Can you work these out from the model? Positions are in its coordinate system, mm. A direction names the side the tool comes from. Round coordinates to 2 decimals unless told otherwise and drop trailing zeros. Order: outer loops, then holes, each group sorted by start corner. A loop starts at its lowest first (then second) coordinate and runs counter-clockwise, first axis right, second up.
from build123d import *

# Parameters (mm, degrees)
SKETCH1_W                    = 25
SKETCH1_H                    = 30
BASE_FLANGE1_DEPTH           = 1.5
EDGE_FLANGE1_STRIP_CUT_DEPTH = 25
EDGE_FLANGE1_DEPTH           = 25
EDGE_FLANGE2_STRIP_CUT_DEPTH = 25
EDGE_FLANGE2_DEPTH           = 25
EDGE_FLANGE3_DEPTH           = 10
EDGE_FLANGE4_DEPTH           = 25
EDGE_FLANGE4_BEND_DEPTH      = 25


# Sheet-metal steps are written as plain solids
with BuildPart() as part:
    # Sketch1 → Base-Flange1 (new body)
    with BuildSketch(Plane(origin=(0, 0, 0), x_dir=(0, 0, -1), z_dir=(1, 0, 0))):
        Rectangle(SKETCH1_W, SKETCH1_H)
    extrude(amount=BASE_FLANGE1_DEPTH)

    # Edge-Flange1 strip (across the edge) → Edge-Flange1 strip cut (cut)
    with BuildSketch(Plane(origin=(1.5, -15, 12.5), x_dir=(0.9063077870366524, 0.4226182617406943, 0), z_dir=(0, 0, -1))):
        Polygon((-4.44875879, 5.991091638), (-1.290447996, -0.781927716), (0.069013684, -0.148000323), (-3.08929711, 6.625019031), align=None)
    extrude(amount=EDGE_FLANGE1_STRIP_CUT_DEPTH, mode=Mode.SUBTRACT)

    # Edge-Flange1 section (across the edge) → Edge-Flange1 (add)
    with BuildSketch(Plane(origin=(1.5, -15, 12.5), x_dir=(0.9063077870366524, 0.4226182617406943, 0), z_dir=(0, 0, -1))):
        with BuildLine():
            Line((-1.5, 0.163300289), (-1.5, 78.667458006))
            Line((-1.5, 78.667458006), (0, 78.667458006))
            Line((0, 78.667458006), (0, 0.163300289))
            ThreePointArc((0, 0.163300289), (0.017460361, 0.003870869), (0.069013684, -0.148000323))
            Line((0.069013684, -0.148000323), (-1.290447996, -0.781927716))
            ThreePointArc((-1.290447996, -0.781927716), (-1.44698365, -0.320788552), (-1.5, 0.163300289))
        make_face()
    extrude(amount=EDGE_FLANGE1_DEPTH)

    # Edge-Flange2 strip (across the edge) → Edge-Flange2 strip cut (cut)
    with BuildSketch(Plane(origin=(34.746304358, -86.296929777, 12.5), x_dir=(0.5735764363510556, 0.8191520442889852, 0), z_dir=(0, 0, -1))):
        Polygon((-4.936952418, 5.551052423), (-1.200352418, -0.920928625), (0.098685688, -0.170928625), (-3.637914312, 6.301052423), align=None)
    extrude(amount=EDGE_FLANGE2_STRIP_CUT_DEPTH, mode=Mode.SUBTRACT)

    # Edge-Flange2 section (across the edge) → Edge-Flange2 (add)
    with BuildSketch(Plane(origin=(34.746304358, -86.296929777, 12.5), x_dir=(0.5735764363510556, 0.8191520442889852, 0), z_dir=(0, 0, -1))):
        with BuildLine():
            Line((-1.5, 0.197371375), (-1.5, 79.598076211))
            Line((-1.5, 79.598076211), (0, 79.598076211))
            Line((0, 79.598076211), (0, 0.197371375))
            ThreePointArc((0, 0.197371375), (0.025099036, 0.006725267), (0.098685688, -0.170928625))
            Line((0.098685688, -0.170928625), (-1.200352418, -0.920928625))
            ThreePointArc((-1.200352418, -0.920928625), (-1.423789703, -0.381503301), (-1.5, 0.197371375))
        make_face()
    extrude(amount=EDGE_FLANGE2_DEPTH)

    # Edge-Flange3 section (across the edge) → Edge-Flange3 (add)
    with BuildSketch(Plane(origin=(100.055624686, -132.027008186, 5), x_dir=(0.2588190451025379, 0.9659258262890636, 0), z_dir=(0, 0, -1))):
        with BuildLine():
            Line((-1.5, 0.129882454), (-1.5, 24.735509529))
            Line((-1.5, 24.735509529), (0, 24.735509529))
            Line((0, 24.735509529), (0, 0.129882454))
            ThreePointArc((0, 0.129882454), (0.011190609, 0.001973206), (0.044422416, -0.122049584))
            Line((0.044422416, -0.122049584), (-1.365116516, -0.635079799))
            ThreePointArc((-1.365116516, -0.635079799), (-1.46602102, -0.25849906), (-1.5, 0.129882454))
        make_face()
    extrude(amount=EDGE_FLANGE3_DEPTH)

    # Edge-Flange4 section (across the edge) → Edge-Flange4 (add)
    with BuildSketch(Plane(origin=(4.738650647, -21.945308726, 12.56444415), x_dir=(0.8925389352890336, 0.41619774072677873, -0.17364817766692378), z_dir=(0.42261826174069417, -0.9063077870366525, 0))):
        with BuildLine():
            Line((-1.5, 0.06444415), (-1.5, 49.868767005))
            Line((-1.5, 49.868767005), (0, 49.868767005))
            Line((0, 49.868767005), (0, 0.06444415))
            ThreePointArc((0, 0.06444415), (0.002802985, 0.000245229), (0.011190609, -0.063465098))
            Line((0.011190609, -0.063465098), (-1.46602102, -0.323937365))
            ThreePointArc((-1.46602102, -0.323937365), (-1.491489062, -0.130488385), (-1.5, 0.06444415))
        make_face()
    extrude(amount=EDGE_FLANGE4_DEPTH)

    # Edge-Flange4 section 2 (across the edge) → Edge-Flange4 bend (add)
    with BuildSketch(Plane(origin=(15.304107191, -44.603003402, -12.56444415), x_dir=(0.8925389352890335, 0.41619774072677895, 0.17364817766692367), z_dir=(-0.4226182617406944, 0.9063077870366524, 0))):
        with BuildLine():
            Line((-1.5, 0.06444415), (-1.5, 49.868767005))
            Line((-1.5, 49.868767005), (0, 49.868767005))
            Line((0, 49.868767005), (0, 0.06444415))
            ThreePointArc((0, 0.06444415), (0.002802985, 0.000245229), (0.011190609, -0.063465098))
            Line((0.011190609, -0.063465098), (-1.46602102, -0.323937365))
            ThreePointArc((-1.46602102, -0.323937365), (-1.491489062, -0.130488385), (-1.5, 0.06444415))
        make_face()
    extrude(amount=EDGE_FLANGE4_BEND_DEPTH)


solid = part.part
(1) I want a section at A-A, the plane z = -10.5. List the corners of the cut face in (x, y) for me.
(2) Please list where these lines run through material, in increasing order: probe 1 along Y at (x, z) = (9.5, 45); probe 2 along X at (y, z) = (-44.5, -9.5); probe 3 along X at (y, z) = (-54, 8.5).
(3) On a 3-axis mill with a long thin cutter (end or side, diameter ignored), from which of +Z, -Z, +X, -X, +Y, -Y can I reach the whole of each face in a straight line? I mean faces 1 (the face through (1.5, 0, 0)), 2 (the face through (17.117, -29.772, 61.808)), 3 (the face through (14.08, -31.57, -37.5)). Say none if no direction works.
(4) I want a section at B-B, the plane y = -123.5. List the corners of the cut face in (x, z) for me, plus the area to 3 significant figures.
(5) I'm going to push flat-ended pins straight in: pin 1 Ø20 at (y, z) = (3.5, 1) entering from +X; pin 2 Ø4 at (x, z) = (14, 11) entering from -Y; pin 3 Ø6.5 at (x, y) = (106, -137) entering from +Z. Where does each tip first touch, or does it pass through?
(6) I want a section at C-C, the plane x = 71. List the corners of the cut face in (y, z) for me.
Ans:
1. outline: (0, -14.84) arc R2.24 ccw to (0.21, -15.78) - (33.3, -86.75) arc R2.24 ccw to (34.05, -87.64) - (99.09, -133.18) - (99.95, -131.95) - (34.91, -86.41) arc R0.74 cw to (34.66, -86.12) - (1.57, -15.15) arc R0.74 cw to (1.5, -14.84) - (1.5, 15) - (0, 15) - close
2. probe 1: y = -22.23 to -19.73
2. probe 2: x = 13.6 to 15.26
2. probe 3: x = 18.03 to 19.69
3. face 1: +Z, -Z, +X, +Y
3. face 2: +Z, +X, +Y
3. face 3: +X, +Y
4. outline: (85.26, -12.5) - (87.88, -12.5) - (87.88, 12.5) - (85.26, 12.5) - close
4. area: 65.4 mm2
5. pin 1: stops at x = 1.5
5. pin 2: stops at y = -49.64
5. pin 3: stops at z = 5
6. outline: (-113.51, -12.5) - (-111.68, -12.5) - (-111.68, 12.5) - (-113.51, 12.5) - close
